```python
from build123d import *

# Parameters (mm, degrees)
F1_DEPTH = 1.5
F2_D     = 4.1
F3_R     = 6
F4_D     = 2.4


with BuildPart() as f1:
    # F0 (on Top) → F1 (new body)
    with BuildSketch(Plane.XY):
        Polygon((155, 99.2472513323), (-126, 99.2472513323), (-126, -91.7527486677), (-1.5, -91.7527486677), (30.5, -91.7527486677), (155, -91.7527486677), align=None)
        with BuildLine():
            ThreePointArc((-76, 61.2472513323), (-74.5355339059, 64.7827852383), (-71, 66.2472513323))
            Line((-71, 66.2472513323), (-41, 66.2472513323))
            ThreePointArc((-41, 66.2472513323), (-37.4644660941, 64.7827852383), (-36, 61.2472513323))
            Line((-36, 61.2472513323), (-36, -53.7527486677))
            ThreePointArc((-36, -53.7527486677), (-37.4644660941, -57.2882825736), (-41, -58.7527486677))
            Line((-41, -58.7527486677), (-71, -58.7527486677))
            ThreePointArc((-71, -58.7527486677), (-74.5355339059, -57.2882825736), (-76, -53.7527486677))
            Line((-76, -53.7527486677), (-76, 61.2472513323))
        make_face(mode=Mode.SUBTRACT)
        with BuildLine():
            Line((105, 61.2472513323), (105, -53.7527486677))
            ThreePointArc((105, -53.7527486677), (103.5355339059, -57.2882825736), (100, -58.7527486677))
            Line((100, -58.7527486677), (70, -58.7527486677))
            ThreePointArc((70, -58.7527486677), (66.4644660941, -57.2882825736), (65, -53.7527486677))
            Line((65, -53.7527486677), (65, 61.2472513323))
            ThreePointArc((65, 61.2472513323), (66.4644660941, 64.7827852383), (70, 66.2472513323))
            Line((70, 66.2472513323), (100, 66.2472513323))
            ThreePointArc((100, 66.2472513323), (103.5355339059, 64.7827852383), (105, 61.2472513323))
        make_face(mode=Mode.SUBTRACT)
    extrude(amount=F1_DEPTH)

    # F2 (through all)
    with Locations(Plane(origin=(0, 0, 0), x_dir=(1, 0, 0), z_dir=(0, 0, -1))):
        with Locations((-114, -87.2472513323), (19, -87.2472513323), (143, 79.7527486677), (-114, 79.7527486677), (19, 79.7527486677)):
            Hole(F2_D / 2)

    # F3
    f3_edges = [f1.edges().sort_by_distance(p)[0] for p in [
        (-126, 99.247251, 0.75),
        (-126, -91.752749, 0.75),
        (155, -91.752749, 0.75),
        (155, 99.247251, 0.75),
    ]]
    fillet(f3_edges, radius=F3_R)

    # F4 (through all)
    with Locations(Plane(origin=(0, 0, 0), x_dir=(1, 0, 0), z_dir=(0, 0, -1))):
        with Locations((-26, -76.2472513323), (-86, -76.2472513323), (-26, 68.7527486677), (-86, 68.7527486677), (55, -76.2472513323), (115, -76.2472513323), (115, 68.7527486677), (55, 68.7527486677)):
            Hole(F4_D / 2)


with BuildPart() as f1_1:
    # F5: moved
    add(f1.part.moved(Location((0, 0, 65))))


with BuildPart() as f1_2:
    # F6: moved
    add(f1_1.part.moved(Location((-2, -2, 0))))


solid = f1_2.part
```
For this review, take the finished solid that the model builds, in its own axes (mm). Round coordinates to 2 decimals unless told otherwise and drop trailing zeros. Order: outer loops, then holes, each group sorted by start corner. A loop starts at its lowest first (then second) coordinate and runs counter-clockwise, first axis right, second up. Notation, with made-up numbers: (53, 7.25) -> (89, 7.25) arc R25 ccw to (89, 29.25) -> close; hole circle Ø7 at (38, 23). An arc over 180 degrees is marked (long way). Use a Markdown table: item, result.
Item 1: Take a section at B-B (y = 34). State the section outline as (x, z) points.
Resolved:
| item | result |
|---|---|
| outline | (-128, 65) -> (-78, 65) -> (-78, 66.5) -> (-128, 66.5) -> close; (-38, 65) -> (63, 65) -> (63, 66.5) -> (-38, 66.5) -> close; (103, 65) -> (153, 65) -> (153, 66.5) -> (103, 66.5) -> close |
Item 2: For line 1 along X through (y, z) = (-8, 66.3); line 2 along X through (y, z) = (-81.5, 65.35); line 3 along Y through (x, z) = (17, 65.4), list the stretches that pass through material, from the lowest coordinate up. Write a range as [from, to].
Resolved:
| item | result |
|---|---|
| line 1 | x = [-128, -78], [-38, 63], [103, 153] |
| line 2 | x = [-128, -118.03], [-113.97, 14.97], [19.03, 138.97], [143.03, 153] |
| line 3 | y = [-93.75, -83.8], [-79.7, 83.2], [87.3, 97.25] |
Item 3: For pin 1 (2 mm diameter, centred on x = -88, y = -70.75, fed in from +Z), flat-tipped, find the tip position at first contact; note if it passes through.
Resolved:
| item | result |
|---|---|
| pin 1 | passes through |
Item 4: Take a section at A-A (x = -65.5). State the section outline as (y, z) points, plus the area to 3 significant figures.
Resolved:
| item | result |
|---|---|
| outline | (-93.75, 65) -> (-60.75, 65) -> (-60.75, 66.5) -> (-93.75, 66.5) -> close; (64.25, 65) -> (97.25, 65) -> (97.25, 66.5) -> (64.25, 66.5) -> close |
| area | 99.0 mm² |
Item 5: Take a section at C-C (z = 65.3). State how many separate pieces and enclosed holes the cut face has, plus the area to 3 significant figures.
Resolved:
| item | result |
|---|---|
| separate pieces | 1 |
| enclosed holes | 15 |
| area | 43,600 mm² |
